Geometry: final body of the model. Coordinates: model frame, mm. A direction names the side the tool comes from. Round coordinates to 2 decimals unless told otherwise and drop trailing zeros. Loops run counter-clockwise (first coordinate to the right, second up) from the corner with the lowest first, then second, coordinate; pieces in that order, holes last. Notation, with made-up numbers: M 60.25,-27.5 L 103.25,-27.5 A14 ccw 103.25,-13.5 Z; hole C -38,20 d9. An arc over 180 degrees is marked long. Return JSON: item names as keys, results as strings.
from build123d import *

# Parameters (mm, degrees)
SKETCH1_R           = 46
BOSS_EXTRUDE1_DEPTH = 20
SKETCH2_R           = 12
BOSS_EXTRUDE2_DEPTH = 10
SKETCH3_R           = 33
CUT_EXTRUDE1_DEPTH  = 14
SKETCH4_R           = 2.5
CUT_EXTRUDE2_DEPTH  = 72.637978754
SKETCH5_R           = 3.5
CUT_EXTRUDE3_DEPTH  = 69.058798109
FILLET1_R           = 1
SKETCH6_R           = 7
CUT_EXTRUDE4_DEPTH  = 10
CHAMFER1_SIZE       = 1
SKETCH8_R           = 4
CUT_EXTRUDE5_DEPTH  = 250


with BuildPart() as part:
    # Sketch1 → Boss-Extrude1 (new body)
    with BuildSketch(Plane(origin=(0, 0, 0), x_dir=(1, 0, 0), z_dir=(0, 1, 0))):
        with Locations(Location((0, 0, 0), (0, 0, 270))):
            Circle(SKETCH1_R)
    extrude(amount=BOSS_EXTRUDE1_DEPTH)

    # Sketch2 → Boss-Extrude2 (add)
    with BuildSketch(Plane.XZ):
        with Locations(Location((0, 0, 0), (0, 0, 270))):
            Circle(SKETCH2_R)
    extrude(amount=BOSS_EXTRUDE2_DEPTH)

    # Sketch3 → Cut-Extrude1 (cut)
    with BuildSketch(Plane(origin=(0, 20, 0), x_dir=(1, 0, 0), z_dir=(0, 1, 0))):
        with Locations(Location((0, 0, 0), (0, 0, 270))):
            Circle(SKETCH3_R)
    extrude(amount=-CUT_EXTRUDE1_DEPTH, mode=Mode.SUBTRACT)

    # Sketch4 → Cut-Extrude2 (cut, through all)
    with BuildSketch(Plane.XZ.offset(10)):
        with Locations(Location((0, 0, 0), (0, 0, 270))):
            Circle(SKETCH4_R)
    extrude(amount=-CUT_EXTRUDE2_DEPTH, mode=Mode.SUBTRACT)

    # Sketch5 → Cut-Extrude3 (cut, through all)
    with BuildSketch(Plane.XZ):
        with Locations(Location((-39, 0, 0), (0, 0, 270))):
            Circle(SKETCH5_R)
        with Locations(Location((-19.5, 33.774990748, 0), (0, 0, 270))):
            Circle(SKETCH5_R)
        with Locations(Location((19.5, 33.774990748, 0), (0, 0, 270))):
            Circle(SKETCH5_R)
        with Locations(Location((39, 0, 0), (0, 0, 270))):
            Circle(SKETCH5_R)
        with Locations(Location((19.5, -33.774990748, 0), (0, 0, 270))):
            Circle(SKETCH5_R)
        with Locations(Location((-19.5, -33.774990748, 0), (0, 0, 270))):
            Circle(SKETCH5_R)
    extrude(amount=-CUT_EXTRUDE3_DEPTH, mode=Mode.SUBTRACT)

    # Fillet1
    fillet1_edges = [part.edges().sort_by_distance(p)[0] for p in [
        (0, 0, -46),
    ]]
    fillet(fillet1_edges, radius=FILLET1_R)

    # Sketch6 → Cut-Extrude4 (cut)
    with BuildSketch(Plane.XZ.offset(10)):
        with Locations(Location((0, 0, 0), (0, 0, 270))):
            Circle(SKETCH6_R)
    extrude(amount=-CUT_EXTRUDE4_DEPTH, mode=Mode.SUBTRACT)

    # Chamfer1
    chamfer1_edges = [part.edges().sort_by_distance(p)[0] for p in [
        (0, -10, 7),
    ]]
    chamfer(chamfer1_edges, length=CHAMFER1_SIZE)

    # Sketch8 → Cut-Extrude5 (cut)
    with BuildSketch(Plane.XY):
        with Locations((0, 12)):
            Circle(SKETCH8_R)
    extrude(amount=-CUT_EXTRUDE5_DEPTH, mode=Mode.SUBTRACT)


solid = part.part
Q1. Reachability of faces 5 (the cylindrical face through (-6.834, -4.563, 1.517)), 6 (the cylindrical face through (-16.55, 9.86, 31.89)), 7 (the cylindrical face through (-12.6, 13.1, 30.5)) from +Z, -Z, +X, -X, +Y, -Y: full face, straight path, thin tool, end or side. Return the list, or none.
Determined:
{"face 5": "-Y", "face 6": "+Y, -Y", "face 7": "+Y"}
Q2. Section query D-D (y = 12). Output: boundary loops of the cut face in (x, z) (3 decimals).
Determined:
{"outline": "M -4,-45.826 L -4,-32.757 A33 cw long 4,-32.757 L 4,-45.826 A46 ccw long Z; hole C -39,0 d7; hole C -19.5,-33.775 d7; hole C -19.5,33.775 d7; hole C 19.5,-33.775 d7; hole C 19.5,33.775 d7; hole C 39,0 d7"}
Q3. Section query C-C (y = -3). Output: boundary loops of the cut face in (x, z).
Determined:
{"outline": "C 0,0 d24; hole C 0,0 d14"}
Q4. Pull-direction query (Y, two-part tool) for faces 1 (the flat face through (-7, 6, 0)), 2 (the cylindrical face through (-0.521, 15.966, -39.286)), 3 (the cylindrical face through (22.45, 9.86, 31.89)), 4 (the flat face through (-9, 0, 9)); classes: pulls with the +Y half, pulls with the -Y half, needs draft (parallel to the pull), parting line crosses it, or undercut.
Determined:
{"face 1": "pulls with the +Y half", "face 2": "undercut", "face 3": "needs draft", "face 4": "pulls with the -Y half"}
Q5. Pin query (flat end, axial travel): pin 1 (3 mm diameter, centred on x = 8, z = -3.5, fed in from +Y); pin 2 (8 mm diameter, centred on x = -19.5, z = -33.77, fed in from -Y); pin 3 (6.5 mm diameter, centred on x = 0, y = 12, fed in from -Z). Return the tip coordinate at first contact, or that it passes through.
Determined:
{"pin 1": "stops at y = 6", "pin 2": "stops at y = 0", "pin 3": "stops at z = 32.84"}
Q6. Section query B-B (y = 3.5). Output: boundary loops of the cut face in (x, z) (3 decimals), plus the area to 3 significant figures.
Determined:
{"outline": "C 0,0 d92; hole C -39,0 d7; hole C -19.5,-33.775 d7; hole C -19.5,33.775 d7; hole C 0,0 d5; hole C 19.5,-33.775 d7; hole C 19.5,33.775 d7; hole C 39,0 d7", "area": "6,400 mm^2"}
Q7. Section query A-A (z = 0). State how many separate pieces and enclosed holes the cut face has, plus the area to 3 significant figures.
Determined:
{"separate pieces": "4", "enclosed holes": "0", "area": "705 mm^2"}
Q8. Material intervals for L1, parallel to X at y = 9.75, z = 0; L2, parallel to X at y = 8, z = 37; L3, parallel to X at y = -5, z = 0, sorted ascending.
Determined:
{"L1": "x = -46 to -42.5, -35.5 to -33, 33 to 35.5, 42.5 to 46", "L2": "x = -27.33 to -20.86, -18.14 to 18.14, 20.86 to 27.33", "L3": "x = -12 to -7, 7 to 12"}
